Verification items for the finished model (mm, model axes). A direction names the side the tool comes from. Round coordinates to 2 decimals unless told otherwise and drop trailing zeros. Loops run counter-clockwise (first coordinate to the right, second up) from the corner with the lowest first, then second, coordinate; pieces in that order, holes last. Notation, with made-up numbers: (-5, 58) -> (40, 58) arc R37 ccw to (40, 97) -> close; hole circle Ø5 at (71.5, -29.5). An arc over 180 degrees is marked (long way). Use a Markdown table: item, result. Add a question column.
```python
from build123d import *

# Parameters (mm, degrees)
SZKIC1_W                    = 12
SZKIC1_H                    = 13
SZKIC1_R                    = 2.25
DODANIE_WYCI_GNI_CIE1_DEPTH = 2
SZKIC2_W                    = 6
SZKIC2_H                    = 13
DODANIE_WYCI_GNI_CIE2_DEPTH = 24
SZKIC3_W                    = 16
SZKIC3_H                    = 13
SZKIC3_R                    = 1.5
DODANIE_WYCI_GNI_CIE3_DEPTH = 2


with BuildPart() as part:
    # Szkic1 → Dodanie-wyciągnięcie1 (new body)
    with BuildSketch(Plane.XY):
        Rectangle(SZKIC1_W, SZKIC1_H)
        with Locations((2.65, 0)):
            Circle(SZKIC1_R, mode=Mode.SUBTRACT)
    extrude(amount=DODANIE_WYCI_GNI_CIE1_DEPTH)

    # Szkic2 → Dodanie-wyciągnięcie2 (add)
    with BuildSketch(Plane.XY.offset(2)):
        with Locations((-3, 0)):
            Rectangle(SZKIC2_W, SZKIC2_H)
    extrude(amount=DODANIE_WYCI_GNI_CIE2_DEPTH)

    # Szkic3 → Dodanie-wyciągnięcie3 (add)
    with BuildSketch(Plane.XY.offset(26)):
        with Locations((-8, 0)):
            Rectangle(SZKIC3_W, SZKIC3_H)
        with Locations((-11, 0)):
            Circle(SZKIC3_R, mode=Mode.SUBTRACT)
    extrude(amount=DODANIE_WYCI_GNI_CIE3_DEPTH)


solid = part.part
```
1) Thickness scan on line 1 (Y direction, x = -11, z = 27.15); line 2 (Y direction, x = 2.65, z = 1.55); line 3 (X direction, y = -4.75, z = 17.75). Record the ranges inside material, lowest first.
2) Sectioned sample at D-D on z = 23.5. Enter the section's corners in (x, y).
3) Access from +Z, -Z, +X, -X, +Y, -Y to the whole of each face (thin tool, end or side, straight path). Record for faces 1 (the face through (5, 2, 2)), 2 (the face through (-6, 0, 13)), 3 (the face through (2.36, 2.23, 0.99)).
4) Go/stop test with flat-tipped pins: pin 1 (3 mm diameter, centred on x = 0.5, y = -4, fed in from -Z); pin 2 (4 mm diameter, centred on y = 4.5, z = 6, fed in from -X); pin 3 (3 mm diameter, centred on x = -9, y = -1, fed in from -Z); pin 4 (6 mm diameter, centred on y = -2, z = 9.5, fed in from +X). Record where each tip stops, or that it passes through.
5) Sectioned sample at C-C on y = -5.5. Enter the section's corners in (x, z), then the cut area to 3 significant figures.
6) Sectioned sample at A-A on y = 0. Enter the section's corners in (x, z), then the cut area to 3 significant figures.
7) Sectioned sample at B-B on x = -11. Enter the section's corners in (y, z), then the cut area to 3 significant figures.
Geometry results:
| question | item | result |
|---|---|---|
| 1 | line 1 | -6.5 to -1.5, 1.5 to 6.5 |
| 1 | line 2 | -6.5 to -2.25, 2.25 to 6.5 |
| 1 | line 3 | -6 to 0 |
| 2 | outline | (-6, -6.5) -> (0, -6.5) -> (0, 6.5) -> (-6, 6.5) -> close |
| 3 | face 1 | +Z, +X, +Y, -Y |
| 3 | face 2 | -Z, -X, +Y, -Y |
| 3 | face 3 | +Z, -Z |
| 4 | pin 1 | z = 0 |
| 4 | pin 2 | x = -6 |
| 4 | pin 3 | z = 26 |
| 4 | pin 4 | x = 0 |
| 5 | outline | (-16, 26) -> (-6, 26) -> (-6, 0) -> (6, 0) -> (6, 2) -> (0, 2) -> (0, 28) -> (-16, 28) -> close |
| 5 | area | 200 mm^2 |
| 6 | outline | (-16, 26) -> (-12.5, 26) -> (-12.5, 28) -> (-16, 28) -> close; (-9.5, 26) -> (-6, 26) -> (-6, 0) -> (0.4, 0) -> (0.4, 2) -> (0, 2) -> (0, 28) -> (-9.5, 28) -> close; (4.9, 0) -> (6, 0) -> (6, 2) -> (4.9, 2) -> close |
| 6 | area | 185 mm^2 |
| 7 | outline | (-6.5, 26) -> (-1.5, 26) -> (-1.5, 28) -> (-6.5, 28) -> close; (1.5, 26) -> (6.5, 26) -> (6.5, 28) -> (1.5, 28) -> close |
| 7 | area | 20.0 mm^2 |
